Read the model definition and answer for the solid it produces. Units are mm, in the model's axes. A direction names the side the tool comes from. Give positions to 0.01 mm unless a question says otherwise; leave off trailing zeros. Order: outer loops, then holes, each group sorted by start corner. A loop starts at its lowest first (then second) coordinate and runs counter-clockwise, first axis right, second up. Notation, with made-up numbers: (50, 46) - (107, 46) arc R21 ccw to (107, 54) - close; hole circle Ø3 at (1, 64.25). An arc over 180 degrees is marked (long way). Return JSON: item names as keys, results as strings.
```python
from build123d import *

# Parameters (mm, degrees)
SKETCH1_W           = 152.4
SKETCH1_H           = 114.3
SKETCH1_R           = 3.175
SKETCH1_R_2         = 2.5
BOSS_EXTRUDE1_DEPTH = 3.175
CUT_EXTRUDE1_REACH  = 158.144
SKETCH2_W           = 35
SKETCH2_H           = 59.5
FILLET1_R           = 3.175
SKETCH4_R           = 2.4892
CUT_EXTRUDE2_DEPTH  = 157.144256218
SKETCH5_R           = 1.8288
CUT_EXTRUDE3_DEPTH  = 157.144256218


with BuildPart() as part:
    # Sketch1 → Boss-Extrude1 (new body)
    with BuildSketch(Plane(origin=(0, 0, 0), x_dir=(1, 0, 0), z_dir=(0, 1, 0))):
        with Locations((69.075, 0)):
            Rectangle(SKETCH1_W, SKETCH1_H)
        with Locations(Location((0, 41.275, 0), (0, 0, 270))):
            Circle(SKETCH1_R, mode=Mode.SUBTRACT)
        with Locations(Location((121.425, 33.75, 0), (0, 0, 270))):
            Circle(SKETCH1_R_2, mode=Mode.SUBTRACT)
        with Locations(Location((138.925, 33.75, 0), (0, 0, 270))):
            Circle(SKETCH1_R_2, mode=Mode.SUBTRACT)
        with Locations(Location((138.925, -33.75, 0), (0, 0, 90))):
            Circle(SKETCH1_R_2, mode=Mode.SUBTRACT)
        with Locations(Location((121.425, -33.75, 0), (0, 0, 90))):
            Circle(SKETCH1_R_2, mode=Mode.SUBTRACT)
        with Locations(Location((0, -41.275, 0), (0, 0, 90))):
            Circle(SKETCH1_R, mode=Mode.SUBTRACT)
        with Locations(Location((57.15, 41.275, 0), (0, 0, 270))):
            Circle(SKETCH1_R, mode=Mode.SUBTRACT)
        with Locations(Location((57.15, -41.275, 0), (0, 0, 90))):
            Circle(SKETCH1_R, mode=Mode.SUBTRACT)
    extrude(amount=BOSS_EXTRUDE1_DEPTH)

    # Sketch2 → Cut-Extrude1 (cut, up to next)
    with BuildSketch(Plane(origin=(0, 3.175, 0), x_dir=(1, 0, 0), z_dir=(0, 1, 0)), mode=Mode.PRIVATE) as cut_extrude1_sk1:
        with Locations((127.775, 0)):
            Rectangle(SKETCH2_W, SKETCH2_H)
    cut_extrude1_tool1 = extrude(cut_extrude1_sk1.sketch, amount=-CUT_EXTRUDE1_REACH, mode=Mode.PRIVATE) & part.part
    # Sketch2 → Cut-Extrude1 (cut, up to next)
    with BuildSketch(Plane(origin=(0, 3.175, 0), x_dir=(1, 0, 0), z_dir=(0, 1, 0)), mode=Mode.PRIVATE) as cut_extrude1_sk2:
        Polygon((-7.125, 0), (-7.125, -31.75), (53.975, -31.75), (53.975, 0), (53.975, 31.75), (-7.125, 31.75), align=None)
    cut_extrude1_tool2 = extrude(cut_extrude1_sk2.sketch, amount=-CUT_EXTRUDE1_REACH, mode=Mode.PRIVATE) & part.part
    add(cut_extrude1_tool1.solids().sort_by_distance((127.775, 3.175, 0))[0], mode=Mode.SUBTRACT)
    add(cut_extrude1_tool2.solids().sort_by_distance((23.425, 3.175, 0))[0], mode=Mode.SUBTRACT)

    # Fillet1
    fillet1_edges = [part.edges().sort_by_distance(p)[0] for p in [
        (110.275, 1.5875, 29.75),
        (110.275, 1.5875, -29.75),
        (53.975, 1.5875, 31.75),
        (53.975, 1.5875, -31.75),
        (145.275, 1.5875, -57.15),
        (145.275, 1.5875, 57.15),
        (-7.125, 1.5875, 57.15),
        (-7.125, 1.5875, -57.15),
    ]]
    fillet(fillet1_edges, radius=FILLET1_R)

    # Sketch4 → Cut-Extrude2 (cut, through all)
    with BuildSketch(Plane(origin=(0, 3.175, 0), x_dir=(1, 0, 0), z_dir=(0, 1, 0))):
        with Locations(Location((72.962713681, 25.4, 0), (0, 0, 270))):
            Circle(SKETCH4_R)
        with Locations(Location((72.962713681, -25.4, 0), (0, 0, 270))):
            Circle(SKETCH4_R)
    extrude(amount=-CUT_EXTRUDE2_DEPTH, mode=Mode.SUBTRACT)

    # Sketch5 → Cut-Extrude3 (cut, through all)
    with BuildSketch(Plane(origin=(0, 3.175, 0), x_dir=(1, 0, 0), z_dir=(0, 1, 0))):
        with Locations(Location((132.575, -47.61738, 0), (0, 0, 270))):
            Circle(SKETCH5_R)
        with Locations(Location((81.775, -47.61738, 0), (0, 0, 270))):
            Circle(SKETCH5_R)
        with Locations(Location((107.175, -47.61738, 0), (0, 0, 270))):
            Circle(SKETCH5_R)
        with Locations(Location((107.175, 47.61738, 0), (0, 0, 90))):
            Circle(SKETCH5_R)
        with Locations(Location((81.775, 47.61738, 0), (0, 0, 90))):
            Circle(SKETCH5_R)
        with Locations(Location((132.575, 47.61738, 0), (0, 0, 90))):
            Circle(SKETCH5_R)
    extrude(amount=-CUT_EXTRUDE3_DEPTH, mode=Mode.SUBTRACT)


solid = part.part
```
Q1. A cutting plane is placed at A-A (x = 57.15). Write down the section's boundary in (y, z) (3 decimals), and give its area (3 significant figures).
Values:
{"outline": "(0, -57.15) - (3.175, -57.15) - (3.175, -44.45) - (0, -44.45) - close; (0, -38.1) - (3.175, -38.1) - (3.175, 38.1) - (0, 38.1) - close; (0, 44.45) - (3.175, 44.45) - (3.175, 57.15) - (0, 57.15) - close", "area": "323 mm²"}
Q2. A cutting plane is placed at C-C (x = 5). Write down the section's boundary in (y, z) (3 decimals).
Values:
{"outline": "(0, -57.15) - (3.175, -57.15) - (3.175, -31.75) - (0, -31.75) - close; (0, 31.75) - (3.175, 31.75) - (3.175, 57.15) - (0, 57.15) - close"}
Q3. Determine the mould class of faces 4 (the cylindrical face through (136.707, 1.565, -32.596)), 5 (the flat face through (68, 0, -1)), 6 (the cylindrical face through (-6.22, 1.61, 56.195)) for opening direction Z: released by +Z, released by -Z, zero draft, split by the parting line, or undercut.
Values:
{"face 4": "undercut", "face 5": "zero draft", "face 6": "released by +Z"}
Q4. Consider L1, parallel to X at y = 1.05, z = 47.5 (3 decimals); L2, parallel to X at y = 0.7, z = -33.75 (3 decimals); L3, parallel to Z at x = 130.5, y = 0.65. Determine where each line is inside the solid, lowest interval first.
Values:
{"L1": "x = -7.125 to 79.95, 83.6 to 105.35, 109 to 130.75, 134.4 to 145.275", "L2": "x = -7.125 to 118.925, 123.925 to 136.425, 141.425 to 145.275", "L3": "z = -57.15 to -29.75, 29.75 to 57.15"}
Q5. For faces 1 (the cylindrical face through (53.07, 1.565, -30.795)), 2 (the flat face through (129, 2, 29.75)), 3 (the cylindrical face through (108.41, 1.61, 46.27)), determine the directions among +Z, -Z, +X, -X, +Y, -Y from which every point of the face is accessible in a straight line to the end or side of a thin tool.
Values:
{"face 1": "-X, +Y, -Y", "face 2": "+X, +Y, -Y", "face 3": "+Y, -Y"}
Q6. A cutting plane is placed at D-D (x = 126). Write down the section's boundary in (y, z) (3 decimals).
Values:
{"outline": "(0, -57.15) - (3.175, -57.15) - (3.175, -29.75) - (0, -29.75) - close; (0, 29.75) - (3.175, 29.75) - (3.175, 57.15) - (0, 57.15) - close"}
Q7. Given pin 1 (1 mm diameter, centred on y = 2.5, z = -3, fed in from +X) (3 decimals); pin 2 (5 mm diameter, centred on x = 0, z = 41.275, fed in from +Y), each flat-ended and moving along its own axis, determine where each tip first touches the part or whether it passes through.
Values:
{"pin 1": "stops at x = 110.275", "pin 2": "passes through"}
Q8. A cutting plane is placed at B-B (z = -33.75). Write down the section's boundary in (x, y) (3 decimals), and give its area (3 significant figures).
Values:
{"outline": "(-7.125, 0) - (118.925, 0) - (118.925, 3.175) - (-7.125, 3.175) - close; (123.925, 0) - (136.425, 0) - (136.425, 3.175) - (123.925, 3.175) - close; (141.425, 0) - (145.275, 0) - (145.275, 3.175) - (141.425, 3.175) - close", "area": "452 mm²"}
